Can you work these out from the model? Positions are in its coordinate system, mm. A direction names the side the tool comes from. Coordinates: 2 decimals unless noted, no trailing zeros. Order: outer loops, then holes, each group sorted by start corner. A loop starts at its lowest first (then second) coordinate and runs counter-clockwise, first axis right, second up. Notation, with made-up numbers: (34.25, -6.75) -> (66.25, -6.75) arc R18 ccw to (66.25, 19.25) -> close; hole circle Ø5 at (-15.75, 38.25). An arc over 180 degrees is marked (long way). Return JSON: item names as keys, results as strings. Group by question number.
1) If we section it at C-C, the plane z = -77: Please give me the cut outline in (x, y).
2) If we section it at A-A, the plane x = 0: Please give me the cut outline in (y, z).
3) If I drill on probe 1 along Z at (x, y) = (1, 3.25); probe 2 along X at (y, z) = (-0.25, -45); probe 3 along Y at (x, z) = (-9.75, -93), over which ranges is the centre line in solid material (lowest first)? Write a range as from..to.
4) Thinking about a two-plate mould opening in Y: for faces 1 (the flat face through (-5, -5, -87)), 2 (the flat face through (0, 8, -100)), 3 (the flat face through (-2, 6, -92)), which applies, +Y half, -Y half, draft (parallel to the pull), parting line (faces both ways), or undercut?
5) For pin 1 (1.5 mm diameter, centred on y = -6, z = -58.5, fed in from -X); pin 2 (5 mm diameter, centred on x = 7, z = -35.5, fed in from +Y); pin 3 (4 mm diameter, centred on y = 9.5, z = -29.5, fed in from -X), each with a flat end and sliding along its axis, tell me the tip position at first contact or that it passes through.
6) If we section it at D-D, the plane x = -9: Please give me the cut outline in (y, z), then the cut area to 3 significant figures.
7) If we section it at B-B, the plane z = -87.5: Please give me the cut outline in (x, y).
8) For faces 4 (the flat face through (0, 0, -74)), 5 (the cylindrical face through (2.5, 8.5, -93.5)), 6 (the cylindrical face through (2.5, -8.5, -93.5)), which set-ups out of +Z, -Z, +X, -X, +Y, -Y let a thin tool reach every point of the face, with its end or its side?
from build123d import *

# Parameters (mm, degrees)
SKETCH_1_R               = 12.5
EXTRUDE_1_DEPTH          = 100
CUT_EXTRUDE_START        = -26
CUT_EXTRUDE_1_DEPTH      = 26
CUT_EXTRUDE_2_DEPTH      = 34
CUT_EXTRUDE_2_DEPTH_BACK = 36.534771414
SKETCH_3_R               = 4.5
SKETCH_6_R               = 6.5
CUT_EXTRUDE_5_DEPTH      = 16


with BuildPart() as part:
    # 스케치1 → 보스-돌출1 (new body)
    with BuildSketch(Plane.XY):
        Circle(SKETCH_1_R)
    extrude(amount=-EXTRUDE_1_DEPTH)

    # 스케치2 → 컷-돌출1 (cut)
    with BuildSketch(Plane(origin=(0, 0, -100), x_dir=(-1, 0, 0), z_dir=(0, 0, -1)).offset(CUT_EXTRUDE_START)):
        with BuildLine():
            Line((11.456439237, 5), (-11.456439237, 5))
            ThreePointArc((-11.456439237, 5), (-12.5, 0), (-11.456439237, -5))
            Line((-11.456439237, -5), (11.456439237, -5))
            ThreePointArc((11.456439237, -5), (12.5, 0), (11.456439237, 5))
        make_face()
    extrude(amount=CUT_EXTRUDE_1_DEPTH, mode=Mode.SUBTRACT)

    # 스케치3 → 컷-돌출2 (cut, two sides: drawn at the far end of the back side and taken through both)
    with BuildSketch(Plane(origin=(0, 0, 0), x_dir=(1, 0, 0), z_dir=(0, 1, 0)).offset(-CUT_EXTRUDE_2_DEPTH_BACK)):
        with Locations(Location((0, 87.5, 0), (0, 0, 90))):
            Circle(SKETCH_3_R)
    extrude(amount=CUT_EXTRUDE_2_DEPTH + CUT_EXTRUDE_2_DEPTH_BACK, mode=Mode.SUBTRACT)

    # 스케치6 → 컷-돌출5 (cut)
    with BuildSketch(Plane(origin=(0, 6, 0), x_dir=(1, 0, 0), z_dir=(0, 1, 0))):
        with Locations(Location((0, 87.5, 0), (0, 0, 90))):
            Circle(SKETCH_6_R)
    cut_extrude_5 = extrude(amount=CUT_EXTRUDE_5_DEPTH, mode=Mode.SUBTRACT)

    # 대칭 복사1: 컷-돌출5 across plane
    add(cut_extrude_5.mirror(Plane.ZX), mode=Mode.SUBTRACT)


solid = part.part
Result sheet:
{
 "1": {"outline": "(-11.46, -5) arc R12.5 ccw to (11.46, -5) -> close; (-11.46, 5) -> (11.46, 5) arc R12.5 ccw to start"},
 "2": {"outline": "(-12.5, -100) -> (-5, -100) -> (-5, -92) -> (-6, -92) -> (-6, -94) -> (-12.5, -94) -> close; (-12.5, -81) -> (-6, -81) -> (-6, -83) -> (-5, -83) -> (-5, -74) -> (5, -74) -> (5, -83) -> (6, -83) -> (6, -81) -> (12.5, -81) -> (12.5, 0) -> (-12.5, 0) -> close; (5, -100) -> (12.5, -100) -> (12.5, -94) -> (6, -94) -> (6, -92) -> (5, -92) -> close"},
 "3": {"probe 1": "z = -74..0", "probe 2": "x = -12.5..12.5", "probe 3": "y = -7.82..-5, 5..7.82"},
 "4": {"face 1": "undercut", "face 2": "draft", "face 3": "+Y half"},
 "5": {"pin 1": "stops at x = -11.34", "pin 2": "stops at y = 11.66", "pin 3": "stops at x = -10"},
 "6": {"outline": "(-8.67, -100) -> (-5, -100) -> (-5, -74) -> (5, -74) -> (5, -100) -> (8.67, -100) -> (8.67, 0) -> (-8.67, 0) -> close", "area": "1,470 mm2"},
 "7": {"outline": "(-11.46, -5) arc R12.5 ccw to (-6.5, -10.68) -> (-6.5, -6) -> (-4.5, -6) -> (-4.5, -5) -> close; (-11.46, 5) -> (-4.5, 5) -> (-4.5, 6) -> (-6.5, 6) -> (-6.5, 10.68) arc R12.5 ccw to start; (4.5, -6) -> (6.5, -6) -> (6.5, -10.68) arc R12.5 ccw to (11.46, -5) -> (4.5, -5) -> close; (4.5, 5) -> (11.46, 5) arc R12.5 ccw to (6.5, 10.68) -> (6.5, 6) -> (4.5, 6) -> close"},
 "8": {"face 4": "-Z, +X, -X", "face 5": "+Y", "face 6": "-Y"}
}
